```python
from build123d import *

# Parameters (mm, degrees)
SKETCH1_W                        = 100
SKETCH1_H                        = 40
BOSS_EXTRUDE1_DEPTH              = 10
SKETCH2_W                        = 50
SKETCH2_H                        = 7.3
BOSS_EXTRUDE2_DEPTH              = 50
FILLET1_R                        = 25
F_12_0MM_DOWEL_HOLE1_D           = 12
F_12_0MM_DOWEL_HOLE1_CSINK_D     = 12.05
F_12_0MM_DOWEL_HOLE1_CSINK_ANGLE = 90
F_5_0MM_DOWEL_HOLE1_D            = 5
F_5_0MM_DOWEL_HOLE1_CSINK_D      = 5.05
F_5_0MM_DOWEL_HOLE1_CSINK_ANGLE  = 90
FILLET2_R                        = 10
FILLET3_R                        = 5


with BuildPart() as part:
    # Sketch1 → Boss-Extrude1 (new body)
    with BuildSketch(Plane(origin=(0, 0, 0), x_dir=(0, 1, 0), z_dir=(0, 0, 1))):
        Rectangle(SKETCH1_W, SKETCH1_H)
    extrude(amount=-BOSS_EXTRUDE1_DEPTH)

    # Sketch2 → Boss-Extrude2 (add)
    with BuildSketch(Plane(origin=(0, 0, 0), x_dir=(0, 1, 0), z_dir=(0, 0, 1))):
        with Locations((0, 16.35)):
            Rectangle(SKETCH2_W, SKETCH2_H)
        with Locations((0, -16.35)):
            Rectangle(SKETCH2_W, SKETCH2_H)
    extrude(amount=BOSS_EXTRUDE2_DEPTH)

    # Fillet1
    fillet1_edges = [part.edges().sort_by_distance(p)[0] for p in [
        (16.35, 25, 50),
        (16.35, -25, 50),
        (-16.35, 25, 50),
        (-16.35, -25, 50),
    ]]
    fillet(fillet1_edges, radius=FILLET1_R - 0.0001)  # a hair under: the kernel refuses the full size

    # Ø12.0mm Dowel Hole1 (through all)
    with Locations(Plane.YZ.offset(20)):
        with Locations((0, 25)):
            CounterSinkHole(F_12_0MM_DOWEL_HOLE1_D / 2, F_12_0MM_DOWEL_HOLE1_CSINK_D / 2, counter_sink_angle=F_12_0MM_DOWEL_HOLE1_CSINK_ANGLE)

    # Ø5.0mm Dowel Hole1 (through all)
    with Locations(Plane(origin=(0, 0, 0), x_dir=(0, 1, 0), z_dir=(0, 0, 1))):
        with Locations((37.5, -15), (-37.5, 15), (-37.5, -15), (37.5, 15)):
            CounterSinkHole(F_5_0MM_DOWEL_HOLE1_D / 2, F_5_0MM_DOWEL_HOLE1_CSINK_D / 2, counter_sink_angle=F_5_0MM_DOWEL_HOLE1_CSINK_ANGLE)

    # Fillet2
    fillet2_edges = [part.edges().sort_by_distance(p)[0] for p in [
        (-20, -50, -5),
        (-20, 50, -5),
        (20, 50, -5),
        (20, -50, -5),
    ]]
    fillet(fillet2_edges, radius=FILLET2_R)

    # Fillet3
    fillet3_edges = [part.edges().sort_by_distance(p)[0] for p in [
        (-16.35, -25, 0),
        (-16.35, 25, 0),
        (16.35, -25, 0),
        (16.35, 25, 0),
    ]]
    fillet(fillet3_edges, radius=FILLET3_R)


solid = part.part
```
Geometry check sheet. Reference: the model listing, model coordinates, mm. A direction names the side the tool comes from. Coordinates: 2 decimals unless noted, no trailing zeros. Loops run counter-clockwise (first coordinate to the right, second up) from the corner with the lowest first, then second, coordinate; pieces in that order, holes last.
Item 1: Sectioned sample at B-B, the plane x = 15. Count the separate pieces of the cut face and the enclosed holes in it, then the cut area to 3 significant figures.
Item 2: Release check for a two-part mould opening along Y. For faces 1 (the face through (0, -1, -10)), 2 (the face through (15.96, 35.19, -5.08)), 3 (the face through (0, -50, -5)) record: released by +Y, released by -Y, zero draft, split by the parting line, or undercut.
Item 3: Go/stop test with flat-tipped pins: pin 1 Ø6.5 at (x, y) = (15, -37.5) entering from -Z; pin 2 Ø8 at (x, y) = (-13, 13) entering from +Z; pin 3 Ø2 at (x, z) = (-16, 15.5) entering from -Y; pin 4 Ø3.5 at (x, z) = (-15.5, 12.5) entering from +Y. Record where each tip stops, or that it passes through.
Item 4: Thickness scan on line 1 (X direction, y = 37.5, z = -3.25); line 2 (X direction, y = -10, z = 36); line 3 (Y direction, x = 15, z = -4). Record the ranges inside material, lowest first.
Item 5: Sectioned sample at A-A, the plane y = 37.5. Record the boundary of the cut face in (x, z) (3 decimals).
Item 6: Sectioned sample at D-D, the plane z = -4.5. Record the boundary of the cut face in (x, y), then the cut area to 3 significant figures.
Item 7: Sectioned sample at C-C, the plane z = 12. Record the boundary of the cut face in (x, y).
Item 8: Access from +Z, -Z, +X, -X, +Y, -Y to the whole of each face (thin tool, end or side, straight path). Record for faces 4 (the face through (16, -25, 15)), 5 (the face through (16, 25, 15)), 6 (the face through (17.15, -46.99, -5.07)).
Check result:
1. separate pieces: 3
1. enclosed holes: 1
1. area: 3,000 mm2
2. face 1: zero draft
2. face 2: undercut
2. face 3: released by -Y
3. pin 1: stops at z = -10
3. pin 2: stops at z = 48.32
3. pin 3: stops at y = -25
3. pin 4: stops at y = 25
4. line 1: x = -20 to -17.5, -12.5 to 12.5, 17.5 to 20
4. line 2: x = -20 to -12.7, 12.7 to 20
4. line 3: y = -48.66 to -40, -35 to 35, 40 to 48.66
5. outline: (-20, -10) - (-17.5, -10) - (-17.5, -0.025) - (-17.525, 0) - (-20, 0) - close; (-12.5, -10) - (12.5, -10) - (12.5, -0.025) - (12.475, 0) - (-12.475, 0) - (-12.5, -0.025) - close; (17.5, -10) - (20, -10) - (20, 0) - (17.525, 0) - (17.5, -0.025) - close
6. outline: (-20, -40) arc R10 ccw to (-10, -50) - (10, -50) arc R10 ccw to (20, -40) - (20, 40) arc R10 ccw to (10, 50) - (-10, 50) arc R10 ccw to (-20, 40) - close; hole circle Ø5 at (-15, -37.5); hole circle Ø5 at (-15, 37.5); hole circle Ø5 at (15, -37.5); hole circle Ø5 at (15, 37.5)
6. area: 3,840 mm2
7. outline: (-20, -25) - (-12.7, -25) - (-12.7, 25) - (-20, 25) - close; (12.7, -25) - (20, -25) - (20, 25) - (12.7, 25) - close
8. face 4: +Z, +X, -X, -Y
8. face 5: +Z, +X, -X, +Y
8. face 6: +Z, -Z, +X, -Y
